Autodesk Inventor part; units mm, degrees
ref_plane "YZ Plane" through (0, 0, 0) normal (1, 0, 0) x (0, 1, 0)
ref_plane "XZ Plane" through (0, 0, 0) normal (0, 1, 0) x (-1, 0, 0)
ref_plane "XY Plane" through (0, 0, 0) normal (0, 0, 1) x (1, 0, 0)
sketch "Sketch1" plane through (0, 0, 0) normal (0, 0, 1) x (1, 0, 0)
  line L0 (0, 0) -> (127, 0)
  line L1 (127, 0) -> (127, 50.8)
  line L2 (127, 50.8) -> (0, 50.8)
  line L3 (0, 50.8) -> (0, 0)
  dimension "d0" = 127
  dimension "d1" = 50.8
extrude "Extrusion1" add sketch "Sketch1" along normal blind 25.4
sketch "Sketch2" plane through (127, 0, 0) normal (1, 0, 0) x (0, 0, -1)
  line L0 (-22.225, 3.175) -> (-3.175, 3.175)
  line L1 (-3.175, 3.175) -> (-3.175, 47.625)
  line L2 (-3.175, 47.625) -> (-22.225, 47.625)
  line L3 (-22.225, 47.625) -> (-22.225, 3.175)
  dimension "d4" = 19.05
  dimension "d5" = 44.45
extrude "Extrusion2" cut sketch "Sketch2" against normal blind 2514.6
sketch "Sketch3" plane through (0, 0, 25.4) normal (0, 0, 1) x (1, 0, 0)
  line L0 (127, 0) -> (127, 50.8)
  line L1 (127, 50.8) -> (0, 50.8)
  line L2 (0, 50.8) -> (0, 0)
  line L3 (0, 0) -> (29.3294, 50.8)
  line L4 (0, 0) -> (58.6588, 0) construction
  line L5 (127, 0) -> (97.6706, 50.8)
  line L6 (127, 0) -> (185.6588, 0) construction
  dimension "d8" = 60
  dimension "d9" = 120
extrude "Extrusion3" cut sketch "Sketch3" against normal blind 2514.6
sketch "Sketch4" plane through (0, 0, 0) normal (0, -1, 0) x (1, 0, 0)
  circle A0 centre (12.7, 12.7) radius 3.175
  circle A1 centre (114.3, 12.7) radius 3.175
  dimension "d12" = 6.35
  dimension "d13" = 6.35
extrude "Extrusion4" cut sketch "Sketch4" against normal blind 2514.6
sketch "Sketch5" plane through (0, 0, 25.4) normal (0, 0, 1) x (1, 0, 0)
  line L0 (0, 0) -> (127, 0)
  line L1 (29.3294, 50.8) -> (97.6706, 50.8)
  line L2 (97.6706, 50.8) -> (97.6706, 0)
  line L3 (97.6706, 0) -> (29.3294, 0)
  line L4 (29.3294, 0) -> (29.3294, 50.8)
  line L5 (29.3294, 0) -> (35.6794, 0)
  line L6 (35.6794, 0) -> (35.6794, 22.2377)
  line L7 (35.6794, 22.2377) -> (97.6706, 22.2377)
  line L8 (97.6706, 22.2377) -> (84.9706, 22.2377)
  circle A0 centre (35.6794, 22.2377) radius 3.175
  dimension "d16" = 6.35
  dimension "d17" = 22.2377
  dimension "d18" = 90
  dimension "d19" = 12.7
  dimension "d20" = 6.35
extrude "Extrusion5" cut sketch "Sketch5" against normal blind 2514.6 contours A0 L7 L6 | L6 L7 A0
properties part number "MotorSupport"
Build history of the part. All positions in model axes, mm. A direction names the side the tool comes from. Give positions to 0.01 mm unless a question says otherwise; leave off trailing zeros. Loops run counter-clockwise (first coordinate to the right, second up) from the corner with the lowest first, then second, coordinate; pieces in that order, holes last. Notation, with made-up numbers: (-25, 67.25) -> (34, 67.25) arc R13 cw to (34, 75.25) -> close; hole circle Ø8 at (3.5, 79.5). An arc over 180 degrees is marked (long way). One line per question, with ' | ' between items. Start each with the question number.
1) Probe L1, parallel to Y at x = 71, z = 10.25 (3 decimals); L2, parallel to Z at x = 69, y = 17 (3 decimals); L3, parallel to Z at x = 12.7, y = 2.1 (3 decimals). List the from-to ranges inside material, lowest first.
2) Cut at A-A (z = 6.5). Give the cut face in (x, y) (3 decimals).
3) Cut at D-D (y = 4.5). Give the cut face in (x, z) (3 decimals).
4) Pin check, flat tips, straight feed: pin 1 (8.5 mm diameter, centred on x = 114.3, z = 12.7, fed in from +Y) (3 decimals); pin 2 (6 mm diameter, centred on y = 43, z = 3.5, fed in from +X); pin 3 (10 mm diameter, centred on y = 17.5, z = 5, fed in from +X). Stop position of each tip, or through.
5) Two-plate mould, pull along X, no slides. Class faces 1 (the cylindrical face through (10.18, 1.57, 10.77)), 2 (the flat face through (112.404, 25.281, 23.107)), 3 (the flat face through (63, 26, 0)): released by +X, released by -X, zero draft, split by the parting line, or undercut.
6) 3-axis set-ups, long thin cutter, end or side, ignore diameter. For faces 4 (the flat face through (64, 50.8, 13)), 5 (the flat face through (64, 25, 3.175)): which of +Z, -Z, +X, -X, +Y, -Y reach the whole face in a straight line?
7) Cut at C-C (z = 12.7). Give the cut face in (x, y) (3 decimals), plus the area to 3 significant figures.
8) Cut at B-B (x = 90). Give the cut face in (y, z) (3 decimals).
Return value:
1) L1: 0 to 3.175, 47.625 to 50.8 | L2: 0 to 3.175, 22.225 to 25.4 | L3: 0 to 9.525, 15.875 to 25.4
2) outline: (0, 0) -> (127, 0) -> (125.167, 3.175) -> (1.833, 3.175) -> close; (27.496, 47.625) -> (99.504, 47.625) -> (97.671, 50.8) -> (29.329, 50.8) -> close
3) outline: (2.598, 0) -> (124.402, 0) -> (124.402, 3.175) -> (2.598, 3.175) -> close; (2.598, 22.225) -> (124.402, 22.225) -> (124.402, 25.4) -> (2.598, 25.4) -> close
4) pin 1: y = 3.175 | pin 2: x = 103.9 | pin 3: x = 119.58
5) face 1: undercut | face 2: released by +X | face 3: zero draft
6) face 4: +Z, -Z, +X, -X, +Y | face 5: +X, -X
7) outline: (0, 0) -> (9.525, 0) -> (9.525, 3.175) -> (1.833, 3.175) -> close; (15.875, 0) -> (111.125, 0) -> (111.125, 3.175) -> (15.875, 3.175) -> close; (27.496, 47.625) -> (99.504, 47.625) -> (97.671, 50.8) -> (29.329, 50.8) -> close; (117.475, 0) -> (127, 0) -> (125.167, 3.175) -> (117.475, 3.175) -> close | area: 580 mm^2
8) outline: (0, 0) -> (50.8, 0) -> (50.8, 25.4) -> (0, 25.4) -> close; hole (3.175, 3.175) -> (47.625, 3.175) -> (47.625, 22.225) -> (3.175, 22.225) -> close
